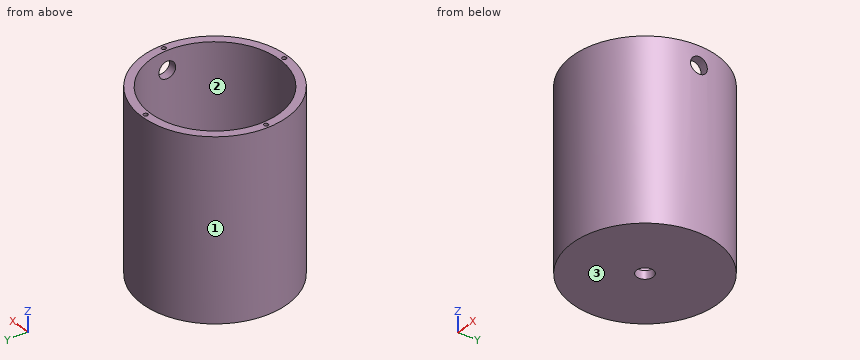
from build123d import *

# Parameters (mm, degrees)
F0_R      = 35
F1_DEPTH  = 86
F2_R      = 31
F3_DEPTH  = 82
F4_R      = 4
F5_DEPTH  = 4
F6_R      = 1
F7_DEPTH  = 4
F9_R      = 4
F10_DEPTH = 4.2601478021


with BuildPart() as f1:
    # F0 (on Top) → F1 (new body)
    with BuildSketch(Plane.XY):
        Circle(F0_R)
    extrude(amount=F1_DEPTH)

    # F2 (on face) → F3 (cut)
    with BuildSketch(Plane.XY.offset(86)):
        Circle(F2_R)
    extrude(amount=-F3_DEPTH, mode=Mode.SUBTRACT)

    # F4 (on face) → F5 (cut, through all)
    with BuildSketch(Plane(origin=(0, 0, 0), x_dir=(1, 0, 0), z_dir=(0, 0, -1))):
        Circle(F4_R)
    extrude(amount=-F5_DEPTH, mode=Mode.SUBTRACT)

    # F6 (on face) → F7 (cut)
    with BuildSketch(Plane.XY.offset(86)):
        with Locations((0, 33)):
            Circle(F6_R)
        with Locations((-33, 0)):
            Circle(F6_R)
        with Locations((0, -33)):
            Circle(F6_R)
        with Locations((33, 0)):
            Circle(F6_R)
    extrude(amount=-F7_DEPTH, mode=Mode.SUBTRACT)

    # F9 (on offset) → F10 (cut, through all)
    with BuildSketch(Plane.YZ.offset(35)):
        with Locations((0, 77)):
            Circle(F9_R)
    extrude(amount=-F10_DEPTH, mode=Mode.SUBTRACT)


solid = f1.part
Build history of the part. All positions in model axes, mm. Face numbers are marked on the shaded views. Round coordinates to 2 decimals unless told otherwise and drop trailing zeros. Loops run counter-clockwise (first coordinate to the right, second up) from the corner with the lowest first, then second, coordinate; pieces in that order, holes last. Notation, with made-up numbers: (9, 19.25) -> (27, 19.25) arc R21 ccw to (27, 42.25) -> close; hole circle Ø2 at (-30.5, 63.5). An arc over 180 degrees is marked (long way). Use CSV: the item, a comma, the result in double quotes. Start each with the question number.
Q1. Mould opens along Y. For the marked faces 1, 2 and 3 say: +Y half, -Y half, draft (parallel to the pull), parting line (faces both ways), or undercut.
Q2. Saw through at C-C on z = 32. Give the cut face in (x, y).
Q3. Saw through at B-B on x = -6. Give the cut face in (y, z), and give its area (3 significant figures).
Q4. Drill centre lines: L1, parallel to Y at x = 0, z = 83; L2, parallel to Y at x = 0, z = 58; L3, parallel to Z at x = -7.5, y = 13. Where is each one in solid material? Low to high.
Q5. Flat gauge pins, fed straight in: pin 1 Ø5 at (y, z) = (0, 77) entering from +X; pin 2 Ø12 at (x, z) = (-0.5, 16) entering from -Y; pin 3 Ø10 at (y, z) = (-15, 40.5) entering from -X. Where does each tip first touch, or does it go through?
Q6. Saw through at A-A on y = 14.5. Give the cut face in (x, z), and give its area (3 significant figures).
Q7. Saw through at D-D on z = 77. Give the cut face in (x, y), and give its area (3 significant figures).
Solutions:
1,face 1,"parting line"
1,face 2,"undercut"
1,face 3,"draft"
2,outline,"circle Ø70 at (0, 0); hole circle Ø62 at (0, 0)"
3,outline,"(-34.48, 0) -> (34.48, 0) -> (34.48, 86) -> (30.41, 86) -> (30.41, 4) -> (-30.41, 4) -> (-30.41, 86) -> (-34.48, 86) -> close"
3,area,"943 mm^2"
4,L1,"y = -35 to -34, -32 to -31, 31 to 32, 34 to 35"
4,L2,"y = -35 to -31, 31 to 35"
4,L3,"z = 0 to 4"
5,pin 1,"stops at x = -30.9"
5,pin 2,"stops at y = -35"
5,pin 3,"stops at x = -33.54"
6,outline,"(-31.86, 0) -> (31.86, 0) -> (31.86, 86) -> (27.4, 86) -> (27.4, 4) -> (-27.4, 4) -> (-27.4, 86) -> (-31.86, 86) -> close"
6,area,"986 mm^2"
7,outline,"(30.74, -4) arc R31 cw (long way) to (30.74, 4) -> (34.77, 4) arc R35 ccw (long way) to (34.77, -4) -> close"
7,area,"797 mm^2"
